CAD build for the part. Positions are in the model's coordinates, mm. A direction names the side the tool comes from. Coordinates: 2 decimals unless noted, no trailing zeros. Order: outer loops, then holes, each group sorted by start corner. A loop starts at its lowest first (then second) coordinate and runs counter-clockwise, first axis right, second up. Notation, with made-up numbers: (-9.5, 76.25) - (22.5, 76.25) arc R8 cw to (22.5, 84.25) - close; hole circle Ø3 at (-2, 28). An arc over 180 degrees is marked (long way). Use one line per item in the form item = value.
```python
from build123d import *

# Parameters (mm, degrees)
F0_R            = 76.2
F1_DEPTH        = 12.7
F3_D            = 12
F3_COPIES_COUNT = 6
F4_R            = 39.8145
F5_DEPTH        = 6.35


# Not quite as in the source:
# - a pattern or mirror of a feature is missing from the dataset's text; its kind, count and spacing are read off the source's solid


with BuildPart() as f1:
    # F0 (on Top) → F1 (new body)
    with BuildSketch(Plane.XY):
        Circle(F0_R)
    extrude(amount=F1_DEPTH)

    # F3 (through all)
    with Locations(Plane.XY.offset(12.7)):
        with Locations((-65, 0)):
            f3 = Hole(F3_D / 2)

    # F3_copies: F3 ×6 about axis
    f3_copies_axis = Axis((0, 0, 0), (0, 0, 1))
    for i in range(1, F3_COPIES_COUNT):
        add(f3.rotate(f3_copies_axis, i * 360 / F3_COPIES_COUNT), mode=Mode.SUBTRACT)

    # F4 (on face) → F5 (cut)
    with BuildSketch(Plane.XY.offset(12.7)):
        Circle(F4_R)
    extrude(amount=-F5_DEPTH, mode=Mode.SUBTRACT)


solid = f1.part
```
Item 1: Two-plate mould, pull along Y, no slides. Class faces 1 (the face through (37.976, 11.959, 9.569)), 2 (the face through (-1, 1, 0)), 3 (the face through (-60.47, -46.367, 6.261)): +Y half, -Y half, draft (parallel to the pull), parting line (faces both ways), or undercut.
Derived:
face_1 = undercut
face_2 = draft
face_3 = parting line
Item 2: Cut at C-C, the plane x = 32.5. Write the cut outline in (y, z).
Derived:
outline = (-68.92, 0) - (-62.29, 0) - (-62.29, 12.7) - (-68.92, 12.7) - close; (-50.29, 0) - (50.29, 0) - (50.29, 12.7) - (23, 12.7) - (23, 6.35) - (-23, 6.35) - (-23, 12.7) - (-50.29, 12.7) - close; (62.29, 0) - (68.92, 0) - (68.92, 12.7) - (62.29, 12.7) - close
Item 3: Cut at B-B, the plane x = 65. Write the cut outline in (y, z).
Derived:
outline = (-39.77, 0) - (-6, 0) - (-6, 12.7) - (-39.77, 12.7) - close; (6, 0) - (39.77, 0) - (39.77, 12.7) - (6, 12.7) - close
Item 4: Drill centre lines: line 1 (Y direction, x = 32.5, z = 9.25); line 2 (Y direction, x = 34.5, z = 9.5); line 3 (Y direction, x = 29, z = 3). Where is each one in solid material? Low to high. Write a range as [from, to].
Derived:
line_1 = [-68.92, -62.29], [-50.29, -23], [23, 50.29], [62.29, 68.92]
line_2 = [-67.94, -61.95], [-50.63, -19.87], [19.87, 50.63], [61.95, 67.94]
line_3 = [-70.47, -61.17], [-51.42, 51.42], [61.17, 70.47]
Item 5: 3-axis set-ups, long thin cutter, end or side, ignore diameter. For faces 4 (the face through (-1, 1, 6.35)), 5 (the face through (-33.281, 50.343, 6.261)): which of +Z, -Z, +X, -X, +Y, -Y reach the whole face in a straight line?
Derived:
face_4 = +Z
face_5 = +Z, -Z
Item 6: Cut at D-D, the plane z = 3.5. Write the cut outline in (x, y).
Derived:
outline = circle Ø152.4 at (0, 0); hole circle Ø12 at (-65, 0); hole circle Ø12 at (-32.5, -56.29); hole circle Ø12 at (-32.5, 56.29); hole circle Ø12 at (32.5, -56.29); hole circle Ø12 at (32.5, 56.29); hole circle Ø12 at (65, 0)
Item 7: Drop flat-ended pins along their axis: pin 1 (4 mm diameter, centred on x = -37, z = 4.5, fed in from +Y); pin 2 (1.5 mm diameter, centred on y = 38.5, z = 7, fed in from -X); pin 3 (1.5 mm diameter, centred on y = -37.5, z = 3, fed in from -X). Give the stop position or say it passes through.
Derived:
pin_1 = 67.69
pin_2 = -66.19
pin_3 = -66.75
Item 8: Cut at A-A, the plane y = 0. Write the cut outline in (x, z).
Derived:
outline = (-76.2, 0) - (-71, 0) - (-71, 12.7) - (-76.2, 12.7) - close; (-59, 0) - (59, 0) - (59, 12.7) - (39.81, 12.7) - (39.81, 6.35) - (-39.81, 6.35) - (-39.81, 12.7) - (-59, 12.7) - close; (71, 0) - (76.2, 0) - (76.2, 12.7) - (71, 12.7) - close
